Verification items for this drawing (mm, ordinates from the low corner). Round coordinates to 2 decimals unless told otherwise and drop trailing zeros. Order: outer loops, then holes, each group sorted by start corner. A loop starts at its lowest first (then second) coordinate and runs counter-clockwise, first axis right, second up. Notation, with made-up numbers: (13, 47.5) -> (50, 47.5) arc R16 ccw to (50, 77.5) -> close; hole circle Ø3 at (82.5, -19). An arc over 180 degrees is marked (long way). Answer in a Markdown table with one row per item. Add a question column.
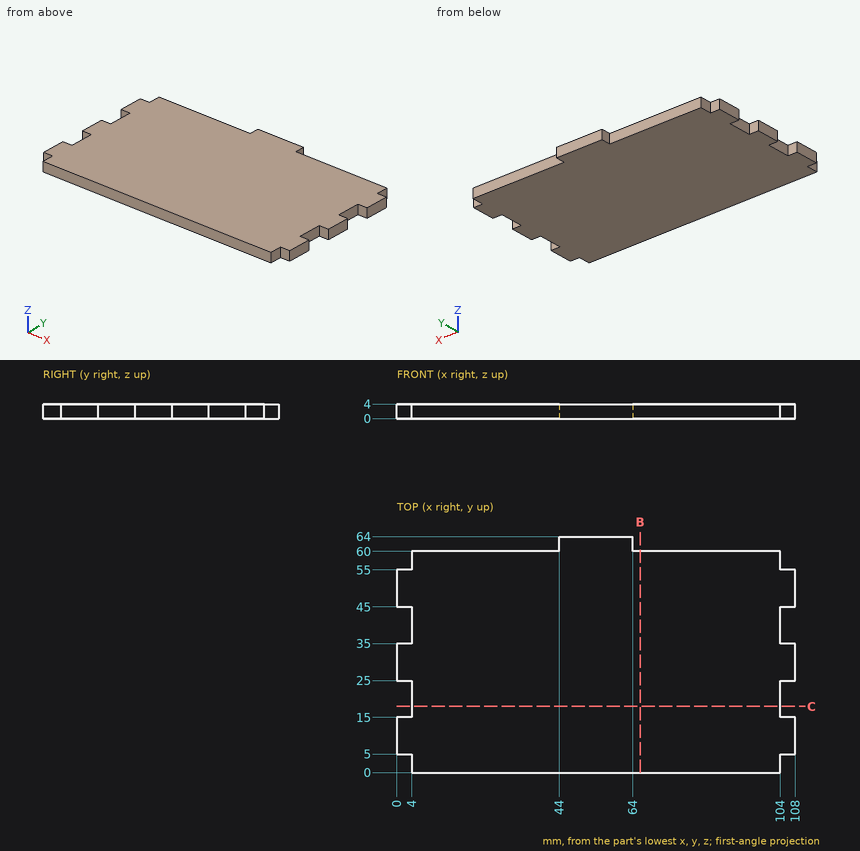
1) Cross-section at B-B, the plane x = 66. Record the boundary of the cut face in (y, z).
2) Depth check by flat-ended pin: P1, Ø1.5, axis at x = 34.5, z = 0.5, coming from the +Y side; P2, Ø1.2, axis at y = 62.5, z = 2.5, coming from the +X side; P3, Ø1.2, axis at x = 106.5, z = 1.5, coming from the +Y side. Enter the tip coordinate at first touch or a pass-through.
3) Cross-section at C-C, the plane y = 18. Record the boundary of the cut face in (x, z), and give its area (3 significant figures).
4) Thickness scan on L1, parallel to X at y = 61.5, z = 2.6; L2, parallel to Y at x = 29, z = 0.6; L3, parallel to X at y = 15.5, z = 2.75. Record the ranges inside material, lowest first. Write a range as [from, to].
Results below:
| question | item | result |
|---|---|---|
| 1 | outline | (0, 0) -> (60, 0) -> (60, 4) -> (0, 4) -> close |
| 2 | P1 | y = 60 |
| 2 | P2 | x = 64 |
| 2 | P3 | y = 55 |
| 3 | outline | (4, 0) -> (104, 0) -> (104, 4) -> (4, 4) -> close |
| 3 | area | 400 mm² |
| 4 | L1 | [44, 64] |
| 4 | L2 | [0, 60] |
| 4 | L3 | [4, 104] |
